from build123d import *

# Parameters (mm, degrees)
BOX587_W                    = 4
BOX587_H                    = 15
BOX587_DEPTH                = 49
CHAMFER054_SIZE             = 3
CHAMFER054_PLACEMENT_ANGLE  = 90
CHAMFER053_SIZE             = 3
CHAMFER053_PLACEMENT_ANGLE  = 135
CHAMFER052_SIZE             = 3
CHAMFER052_PLACEMENT_ANGLE  = 180
CHAMFER051_SIZE             = 3
CHAMFER051_PLACEMENT_ANGLE  = 225
CHAMFER050_SIZE             = 3
CHAMFER050_PLACEMENT_ANGLE  = 90
CHAMFER049_SIZE             = 3
CHAMFER049_PLACEMENT_ANGLE  = 45
CHAMFER056_SIZE             = 3
CHAMFER055_SIZE             = 3
CHAMFER055_PLACEMENT_ANGLE  = 45
COMPOUND992_PLACEMENT_ANGLE = 90
BOX596_W                    = 6
BOX596_H                    = 6
BOX596_DEPTH                = 64
BOX597_W                    = 6
BOX597_H                    = 6
BOX597_DEPTH                = 64
CYLINDER2411_R              = 60.2
CYLINDER2411_DEPTH          = 58
CYLINDER2395_R              = 1.5
CYLINDER2395_DEPTH          = 32
CYLINDER2380_R              = 1.5
CYLINDER2380_DEPTH          = 32
CYLINDER2370_R              = 1.5
CYLINDER2370_DEPTH          = 100
CYLINDER2383_R              = 1.5
CYLINDER2383_DEPTH          = 100
CYLINDER2384_R              = 3
CYLINDER2384_DEPTH          = 3
CYLINDER2387_R              = 3
CYLINDER2387_DEPTH          = 3
CYLINDER2377_R              = 1.5
CYLINDER2377_DEPTH          = 50
CYLINDER2369_R              = 1.5
CYLINDER2369_DEPTH          = 50
CYLINDER2358_R              = 1.5
CYLINDER2358_DEPTH          = 50
CYLINDER2366_R              = 1.5
CYLINDER2366_DEPTH          = 50
CYLINDER2355_R              = 1.5
CYLINDER2355_DEPTH          = 100
CYLINDER2376_R              = 1.5
CYLINDER2376_DEPTH          = 100
CYLINDER2372_R              = 1.5
CYLINDER2372_DEPTH          = 100
CYLINDER2381_R              = 1.5
CYLINDER2381_DEPTH          = 100
BOX591_W                    = 72
BOX591_H                    = 70
BOX591_DEPTH                = 10
CUT583_PLACEMENT_ANGLE      = 180


with BuildPart() as krychle587:
    # Box587 → Box587 (new body)
    with BuildSketch(Plane(origin=(59, -7.5, 20), x_dir=(1, 0, 0), z_dir=(0, 0, 1))):
        with Locations((2, 7.5)):
            Rectangle(BOX587_W, BOX587_H)
    extrude(amount=BOX587_DEPTH)


with BuildPart() as chamfer054:
    # Chamfer054 base: copy of Krychle587
    add(krychle587.part)

    # Chamfer054
    chamfer054_edges = [chamfer054.edges().sort_by_distance(p)[0] for p in [
        (63, -7.5, 44.5),
        (63, 7.5, 44.5),
    ]]
    chamfer(chamfer054_edges, length=CHAMFER054_SIZE)


with BuildPart() as chamfer054_1:
    # Chamfer054 placement: moved
    add(chamfer054.part.rotate(Axis((0, 0, 0), (0, 0, 1)), CHAMFER054_PLACEMENT_ANGLE))


with BuildPart() as chamfer053:
    # Chamfer053 base: copy of Krychle587
    add(krychle587.part)

    # Chamfer053
    chamfer053_edges = [chamfer053.edges().sort_by_distance(p)[0] for p in [
        (63, -7.5, 44.5),
        (63, 7.5, 44.5),
    ]]
    chamfer(chamfer053_edges, length=CHAMFER053_SIZE)


with BuildPart() as chamfer053_1:
    # Chamfer053 placement: moved
    add(chamfer053.part.rotate(Axis((0, 0, 0), (0, 0, 1)), CHAMFER053_PLACEMENT_ANGLE))


with BuildPart() as chamfer052:
    # Chamfer052 base: copy of Krychle587
    add(krychle587.part)

    # Chamfer052
    chamfer052_edges = [chamfer052.edges().sort_by_distance(p)[0] for p in [
        (63, -7.5, 44.5),
        (63, 7.5, 44.5),
    ]]
    chamfer(chamfer052_edges, length=CHAMFER052_SIZE)


with BuildPart() as chamfer052_1:
    # Chamfer052 placement: moved
    add(chamfer052.part.rotate(Axis((0, 0, 0), (0, 0, 1)), CHAMFER052_PLACEMENT_ANGLE))


with BuildPart() as chamfer051:
    # Chamfer051 base: copy of Krychle587
    add(krychle587.part)

    # Chamfer051
    chamfer051_edges = [chamfer051.edges().sort_by_distance(p)[0] for p in [
        (63, -7.5, 44.5),
        (63, 7.5, 44.5),
    ]]
    chamfer(chamfer051_edges, length=CHAMFER051_SIZE)


with BuildPart() as chamfer051_1:
    # Chamfer051 placement: moved
    add(chamfer051.part.rotate(Axis((0, 0, 0), (0, 0, 1)), CHAMFER051_PLACEMENT_ANGLE))


with BuildPart() as chamfer050:
    # Chamfer050 base: copy of Krychle587
    add(krychle587.part)

    # Chamfer050
    chamfer050_edges = [chamfer050.edges().sort_by_distance(p)[0] for p in [
        (63, -7.5, 44.5),
        (63, 7.5, 44.5),
    ]]
    chamfer(chamfer050_edges, length=CHAMFER050_SIZE)


with BuildPart() as chamfer050_1:
    # Chamfer050 placement: moved
    add(chamfer050.part.rotate(Axis((0, 0, 0), (0, 0, -1)), CHAMFER050_PLACEMENT_ANGLE))


with BuildPart() as chamfer049:
    # Chamfer049 base: copy of Krychle587
    add(krychle587.part)

    # Chamfer049
    chamfer049_edges = [chamfer049.edges().sort_by_distance(p)[0] for p in [
        (63, -7.5, 44.5),
        (63, 7.5, 44.5),
    ]]
    chamfer(chamfer049_edges, length=CHAMFER049_SIZE)


with BuildPart() as chamfer049_1:
    # Chamfer049 placement: moved
    add(chamfer049.part.rotate(Axis((0, 0, 0), (0, 0, -1)), CHAMFER049_PLACEMENT_ANGLE))


with BuildPart() as chamfer056:
    # Chamfer056 base: copy of Krychle587
    add(krychle587.part)

    # Chamfer056
    chamfer056_edges = [chamfer056.edges().sort_by_distance(p)[0] for p in [
        (63, -7.5, 44.5),
        (63, 7.5, 44.5),
    ]]
    chamfer(chamfer056_edges, length=CHAMFER056_SIZE)


with BuildPart() as compound992:
    # Chamfer055 base: copy of Krychle587
    add(krychle587.part)

    # Chamfer055
    chamfer055_edges = [compound992.edges().sort_by_distance(p)[0] for p in [
        (63, -7.5, 44.5),
        (63, 7.5, 44.5),
    ]]
    chamfer(chamfer055_edges, length=CHAMFER055_SIZE)


with BuildPart() as compound992_1:
    # Chamfer055 placement: moved
    add(compound992.part.rotate(Axis((0, 0, 0), (0, 0, 1)), CHAMFER055_PLACEMENT_ANGLE))

    # Compound992: union Chamfer054, Chamfer053, Chamfer052, Chamfer051, Chamfer050, Chamfer049, Chamfer056
    add(chamfer054_1.part)
    add(chamfer053_1.part)
    add(chamfer052_1.part)
    add(chamfer051_1.part)
    add(chamfer050_1.part)
    add(chamfer049_1.part)
    add(chamfer056.part)


with BuildPart() as compound992_2:
    # Compound992 placement: moved
    add(compound992_1.part.moved(Location((52, -39, -89))).rotate(Axis((52, -39, -89), (-1, 0, 0)), COMPOUND992_PLACEMENT_ANGLE))


with BuildPart() as krychle596:
    # Box596 → Box596 (new body)
    with BuildSketch(Plane(origin=(87, -3, -93), x_dir=(1, 0, 0), z_dir=(0, 0, 1))):
        with Locations((3, 3)):
            Rectangle(BOX596_W, BOX596_H)
    extrude(amount=BOX596_DEPTH)


with BuildPart() as compound1007:
    # Box597 → Box597 (new body)
    with BuildSketch(Plane(origin=(11, -3, -93), x_dir=(1, 0, 0), z_dir=(0, 0, 1))):
        with Locations((3, 3)):
            Rectangle(BOX597_W, BOX597_H)
    extrude(amount=BOX597_DEPTH)

    # Compound1007: union Krychle596
    add(krychle596.part)


with BuildPart() as compound1007_1:
    # Compound1007 placement: moved
    add(compound1007.part.moved(Location((-52, 0, 36))))


with BuildPart() as obj1:
    # Cylinder2411 → Cylinder2411 (new body)
    with BuildSketch(Plane(origin=(0, 19, -53), x_dir=(1, 0, 0), z_dir=(0, -1, 0))):
        Circle(CYLINDER2411_R)
    extrude(amount=CYLINDER2411_DEPTH)


with BuildPart() as obj2:
    # Cylinder2395 → Cylinder2395 (new body)
    with BuildSketch(Plane(origin=(78, 41, -42), x_dir=(1, 0, 0), z_dir=(0, 0, 1))):
        Circle(CYLINDER2395_R)
    extrude(amount=CYLINDER2395_DEPTH)


with BuildPart() as compound1001:
    # Cylinder2380 → Cylinder2380 (new body)
    with BuildSketch(Plane(origin=(26, 41, -42), x_dir=(1, 0, 0), z_dir=(0, 0, 1))):
        Circle(CYLINDER2380_R)
    extrude(amount=CYLINDER2380_DEPTH)

    # Compound1001: union obj2
    add(obj2.part)


with BuildPart() as compound1001_1:
    # Compound1001 placement: moved
    add(compound1001.part.moved(Location((-52, 0, 36))))


with BuildPart() as obj3:
    # Cylinder2370 → Cylinder2370 (new body)
    with BuildSketch(Plane(origin=(14, 0, -60), x_dir=(1, 0, 0), z_dir=(0, 0, 1))):
        Circle(CYLINDER2370_R)
    extrude(amount=CYLINDER2370_DEPTH)


with BuildPart() as compound1011:
    # Cylinder2383 → Cylinder2383 (new body)
    with BuildSketch(Plane(origin=(90, 0, -60), x_dir=(1, 0, 0), z_dir=(0, 0, 1))):
        Circle(CYLINDER2383_R)
    extrude(amount=CYLINDER2383_DEPTH)

    # Compound1003: union obj3
    add(obj3.part)


with BuildPart() as compound1011_1:
    # Compound1003 placement: moved
    add(compound1011.part.moved(Location((-52, 0, 0))))

    # Compound1011: union Compound1001
    add(compound1001_1.part)


with BuildPart() as obj4:
    # Cylinder2384 → Cylinder2384 (new body)
    with BuildSketch(Plane(origin=(78, 41, -42), x_dir=(1, 0, 0), z_dir=(0, 0, 1))):
        Circle(CYLINDER2384_R)
    extrude(amount=CYLINDER2384_DEPTH)


with BuildPart() as compound1020:
    # Cylinder2387 → Cylinder2387 (new body)
    with BuildSketch(Plane(origin=(26, 41, -42), x_dir=(1, 0, 0), z_dir=(0, 0, 1))):
        Circle(CYLINDER2387_R)
    extrude(amount=CYLINDER2387_DEPTH)

    # Compound1020: union obj4
    add(obj4.part)


with BuildPart() as compound1020_1:
    # Compound1020 placement: moved
    add(compound1020.part.moved(Location((-52, 0, 42))))


with BuildPart() as obj5:
    # Cylinder2377 → Cylinder2377 (new body)
    with BuildSketch(Plane(origin=(-51, 6, 0), x_dir=(1, 0, 0), z_dir=(0, 0, 1))):
        Circle(CYLINDER2377_R)
    extrude(amount=CYLINDER2377_DEPTH)


with BuildPart() as obj6:
    # Cylinder2369 → Cylinder2369 (new body)
    with BuildSketch(Plane(origin=(-24, 18, 0), x_dir=(1, 0, 0), z_dir=(0, 0, 1))):
        Circle(CYLINDER2369_R)
    extrude(amount=CYLINDER2369_DEPTH)


with BuildPart() as obj7:
    # Cylinder2358 → Cylinder2358 (new body)
    with BuildSketch(Plane(origin=(24, 18, 0), x_dir=(1, 0, 0), z_dir=(0, 0, 1))):
        Circle(CYLINDER2358_R)
    extrude(amount=CYLINDER2358_DEPTH)


with BuildPart() as compound998:
    # Cylinder2366 → Cylinder2366 (new body)
    with BuildSketch(Plane(origin=(51, 6, 0), x_dir=(1, 0, 0), z_dir=(0, 0, 1))):
        Circle(CYLINDER2366_R)
    extrude(amount=CYLINDER2366_DEPTH)

    # Compound998: union obj5, obj6, obj7
    add(obj5.part)
    add(obj6.part)
    add(obj7.part)


with BuildPart() as compound998_1:
    # Compound998 placement: moved
    add(compound998.part.moved(Location((0, 6, 0))))


with BuildPart() as obj8:
    # Cylinder2355 → Cylinder2355 (new body)
    with BuildSketch(Plane(origin=(51, -12, 0), x_dir=(1, 0, 0), z_dir=(0, 0, 1))):
        Circle(CYLINDER2355_R)
    extrude(amount=CYLINDER2355_DEPTH)


with BuildPart() as compound1019:
    # Cylinder2376 → Cylinder2376 (new body)
    with BuildSketch(Plane(origin=(-51, -12, 0), x_dir=(1, 0, 0), z_dir=(0, 0, 1))):
        Circle(CYLINDER2376_R)
    extrude(amount=CYLINDER2376_DEPTH)

    # Compound1019: union obj8
    add(obj8.part)


with BuildPart() as obj9:
    # Cylinder2372 → Cylinder2372 (new body)
    with BuildSketch(Plane(origin=(39, -21, 0), x_dir=(1, 0, 0), z_dir=(0, 0, 1))):
        Circle(CYLINDER2372_R)
    extrude(amount=CYLINDER2372_DEPTH)


with BuildPart() as compound995:
    # Cylinder2381 → Cylinder2381 (new body)
    with BuildSketch(Plane(origin=(-39, -21, 0), x_dir=(1, 0, 0), z_dir=(0, 0, 1))):
        Circle(CYLINDER2381_R)
    extrude(amount=CYLINDER2381_DEPTH)

    # Compound1000: union obj9
    add(obj9.part)


with BuildPart() as compound995_1:
    # Compound1000 placement: moved
    add(compound995.part.moved(Location((0, -6, 0))))

    # Compound995: union Compound998, Compound1019
    add(compound998_1.part)
    add(compound1019.part)


with BuildPart() as compound995_2:
    # Compound995 placement: moved
    add(compound995_1.part.moved(Location((0, 0, -10))))


with BuildPart() as cut594:
    # Box591 → Box591 (new body)
    with BuildSketch(Plane(origin=(-36, -30, 0), x_dir=(1, 0, 0), z_dir=(0, 0, 1))):
        with Locations((36, 35)):
            Rectangle(BOX591_W, BOX591_H)
    extrude(amount=BOX591_DEPTH)

    # Cut582: cut Compound995
    add(compound995_2.part, mode=Mode.SUBTRACT)

    # Cut576: cut Compound1020
    add(compound1020_1.part, mode=Mode.SUBTRACT)

    # Cut573: cut Compound1011
    add(compound1011_1.part, mode=Mode.SUBTRACT)

    # Cut579: cut obj1
    add(obj1.part, mode=Mode.SUBTRACT)

    # Cut583: cut Compound1007
    add(compound1007_1.part, mode=Mode.SUBTRACT)


with BuildPart() as cut594_1:
    # Cut583 placement: moved
    add(cut594.part.moved(Location((52, 0, -36))).rotate(Axis((52, 0, -36), (0, 0, 1)), CUT583_PLACEMENT_ANGLE))

    # Cut594: cut Compound992
    add(compound992_2.part, mode=Mode.SUBTRACT)


solid = cut594_1.part
Part model, mm, in its own coordinate system. A direction names the side the tool comes from. Round coordinates to 2 decimals unless told otherwise and drop trailing zeros. Write each loop counter-clockwise with the first axis right and the second up, starting at its lowest first coordinate (ties: lowest second). Pieces come first, ordered by that corner, then holes. Notation, with made-up numbers: (40, -34) - (92, -34) arc R16 cw to (92, -6) - close; hole circle Ø11 at (-25.5, 60). An arc over 180 degrees is marked (long way). Use CSV: the item, a comma, the result in double quotes.
Item 1: Slice it at D-D, the plane x = 28. Write the cut outline in (y, z).
Results list:
outline,"(-40, -33) - (-38.76, -33) - (-38.76, -36) - (-25.5, -36) - (-25.5, -26) - (-40, -26) - close; (-22.5, -36) - (-19, -36) - (-19, -33.79) - (30, -33.79) - (30, -26) - (-22.5, -26) - close"
Item 2: Tool access for faces 5 (the flat face through (17, 0, -33)), 6 (the flat face through (46, 5.2, -27.5)), 7 (the flat face through (78, -39, -33)): list every direction of +Z, -Z, +X, -X, +Y, -Y with a clear straight run to the whole face (end or side of a thin tool).
Results list:
face 5,"-Z, -X"
face 6,"-Z, +Y"
face 7,"-Z, -Y"
Item 3: Wall check: L1, parallel to Y at x = 76, z = -32.5; L2, parallel to X at y = -23, z = -26.5; L3, parallel to Y at x = 53, z = -27. Give the ranges that are in metal, low to high.
Results list:
L1,"y = -40 to -25.5, -22.5 to 30"
L2,"x = 16 to 26.88, 29.12 to 74.88, 77.12 to 88"
L3,"y = -40 to -19"
Item 4: Slice it at C-C, the plane y = -24. Write the cut outline in (x, z).
Results list:
outline,"(16, -36) - (26.5, -36) - (26.5, -26) - (16, -26) - close; (29.5, -36) - (74.5, -36) - (74.5, -26) - (29.5, -26) - close; (77.5, -36) - (88, -36) - (88, -26) - (77.5, -26) - close"
Item 5: Slice it at B-B, the plane z = -27.5. Write the cut outline in (x, y), then the cut area to 3 significant figures.
Results list:
outline,"(16, -40) - (24.88, -40) arc R1.5 cw to (27.12, -40) - (76.88, -40) arc R1.5 cw to (79.12, -40) - (88, -40) - (88, 30) - (58, 30) - (58, -19) - (46, -19) - (46, 30) - (16, 30) - close; hole circle Ø3 at (28, -24); hole circle Ø3 at (76, -24)"
area,"4,440 mm²"
Item 6: Flat gauge pins, fed straight in: P1, Ø1.8, axis at y = 0.5, z = -31, coming from the -X side; P2, Ø2, axis at x = 25.5, y = -39.5, coming from the -Z side; P3, Ø3, axis at x = 50, z = -32, coming from the +Y side; P4, Ø1.8, axis at x = 76, y = -24, coming from the +Z side (3 decimals). Where does each tip first touch, or does it go through?
Results list:
P1,"stops at x = 17"
P2,"stops at z = -33"
P3,"stops at y = -19"
P4,"passes through"
Item 7: Pull direction X, two halves, no side cores. Call faces 1 (the flat face through (84, -40, -31)), 2 (the flat face through (16, -5, -31)), 3 (the cylindrical face through (78, -38, -35)), 4 (the flat face through (26, -39, -33)): pulls with the +X half, pulls with the -X half, needs draft (parallel to the pull), parting line crosses it, or undercut.
Results list:
face 1,"needs draft"
face 2,"pulls with the -X half"
face 3,"undercut"
face 4,"undercut"
Item 8: Slice it at A-A, the plane y = 5. Write the cut outline in (x, z).
Results list:
outline,"(16, -36) - (23.45, -36) arc R60.2 cw to (44.5, -29.27) - (44.5, -29) - (47.5, -26) - (16, -26) - close; (56.5, -26) - (59.5, -29) - (59.5, -29.27) arc R60.2 cw to (80.55, -36) - (88, -36) - (88, -26) - close"
